Verification items for the finished model (mm, model axes). A direction names the side the tool comes from. Give positions to 0.01 mm unless a question says otherwise; leave off trailing zeros. Write each loop counter-clockwise with the first axis right and the second up, starting at its lowest first coordinate (ties: lowest second). Pieces come first, ordered by that corner, then holes. Notation, with made-up numbers: (24, -14) -> (29, -14) arc R26 ccw to (29, 18) -> close; hole circle Ø9 at (84, -29). An arc over 180 degrees is marked (long way). Answer as CSV lines item,"result". Start each with the question number.
1) Material ranges on L1, parallel to Y at x = 0, z = 0.75; L2, parallel to Y at x = -1, z = 1; L3, parallel to Z at x = 8.5, y = 3.5, recorded low to high.
2) Mould release check, pull along Y, two halves, no side actions. Record for faces 4 (the flat face through (3.647, 1.634, 6.234)), 5 (the flat face through (-1.836, -3.251, 3.847)), 6 (the flat face through (4.3, 2.4, 1.5)), 7 (the flat face through (1.836, 3.251, 3.885)): released by +Y, released by -Y, zero draft, split by the parting line, or undercut.
3) Tool access check on faces 1 (the cylindrical face through (-1.177, -3.875, 6.935)), 2 (the cylindrical face through (-3.35, -1.89, 5.49)), 3 (the flat face through (3.251, 1.836, 3.847)). Record the directions out of +Z, -Z, +X, -X, +Y, -Y that give a thin tool (end or side, any length) a straight path to the whole face; none if there is none.
4) Gauge pin test, flat ends, axial feed: pin 1 Ø3.5 at (x, y) = (0, -7) entering from +Z; pin 2 Ø3 at (y, z) = (-4, 1) entering from +X; pin 3 Ø4 at (x, z) = (4.5, 4) entering from +Y. Record the tip position at first contact, or that the pin passes through.
5) Sectioned sample at D-D on y = 7. Record the cut outline in (x, z).
6) Sectioned sample at C-C on z = 2.75. Record the cut outline in (x, y), and give its area (3 significant figures).
7) Sectioned sample at B-B on x = 0. Record the cut outline in (y, z).
8) Sectioned sample at A-A on z = 1. Record the cut outline in (x, y), and give its area (3 significant figures).
```python
from build123d import *

# Parameters (mm, degrees)
ESQUISSE1_R                  = 3
BOSS_EXTRU_1_DEPTH           = 1.5
ENL_V_MAT_EXTRU_1_DEPTH      = 16.779733838
ENL_V_MAT_EXTRU_1_DEPTH_BACK = 16.779733838
ESQUISSE4_R                  = 1.5
ENL_V_MAT_EXTRU_2_DEPTH      = 14.2
CONG_2_R                     = 0.5


with BuildPart() as part:
    # Esquisse1 → Boss.-Extru.1 (new body)
    with BuildSketch(Plane.XY):
        with BuildLine():
            Line((-4.5, 8.93028555), (-4.5, -8.93028555))
            ThreePointArc((-4.5, -8.93028555), (5.029430583, -8.643195475), (9.987487585, -0.500091723))
            ThreePointArc((9.987487585, -0.500091723), (5.455376603, 8.380863089), (-4.5, 8.93028555))
        make_face()
        with Locations(Location((0, 0, 0), (0, 0, 180))):
            Circle(ESQUISSE1_R, mode=Mode.SUBTRACT)
    extrude(amount=BOSS_EXTRU_1_DEPTH)

    # Esquisse2 → R_volution1 (revolve)
    with BuildSketch(Plane(origin=(0, 0, 0), x_dir=(0, 0, -1), z_dir=(1, 0, 0)), mode=Mode.PRIVATE) as r_volution1_sk:
        Polygon((-1.5, 4.5), (-7, 4.5), (-7, 3.669872981), (-4.5, 3), (-1.5, 3), align=None)
    revolve(r_volution1_sk.sketch.rotate(Axis((0, 0, 0), (0, 0, 1)), 90), axis=Axis((0, 0, 0), (0, 0, 1)))

    # Esquisse3 → Enl_v. mat.-Extru.1 (cut, two sides)
    with BuildSketch(Plane(origin=(0, 0, 0), x_dir=(0, 0, 1), z_dir=(0.7071067811865464, 0.7071067811865488, 0))) as enl_v_mat_extru_1_sk:
        with BuildLine():
            Line((2.5, 1), (5.232050808, 1))
            ThreePointArc((5.232050808, 1), (5.490869853, 1.034074174), (5.732050808, 1.133974596))
            Line((5.732050808, 1.133974596), (7, 1.866025404))
            Line((7, 1.866025404), (7, -1.866025404))
            Line((7, -1.866025404), (5.732050808, -1.133974596))
            ThreePointArc((5.732050808, -1.133974596), (5.490869853, -1.034074174), (5.232050808, -1))
            Line((5.232050808, -1), (2.5, -1))
            ThreePointArc((2.5, -1), (1.5, 0), (2.5, 1))
        make_face()
    extrude(amount=ENL_V_MAT_EXTRU_1_DEPTH, mode=Mode.SUBTRACT)
    extrude(enl_v_mat_extru_1_sk.sketch, amount=-ENL_V_MAT_EXTRU_1_DEPTH_BACK, mode=Mode.SUBTRACT)

    # Esquisse4 → Enl_v. mat.-Extru.2 (cut)
    with BuildSketch(Plane.XY.offset(1.5)):
        with Locations((0, -7)):
            Circle(ESQUISSE4_R)
        with Locations((0, 7)):
            Circle(ESQUISSE4_R)
        with Locations((7, 0)):
            Circle(ESQUISSE4_R)
    extrude(amount=-ENL_V_MAT_EXTRU_2_DEPTH, mode=Mode.SUBTRACT)

    # Cong_2
    cong_2_edges = [part.edges().sort_by_distance(p)[0] for p in [
        (-3.884480351, -1.245521917, 7),
        (1.245521917, 3.884480351, 7),
        (3.884480351, 1.245521917, 7),
        (-1.245521917, -3.884480351, 7),
    ]]
    fillet(cong_2_edges, radius=CONG_2_R)


solid = part.part
```
Ans:
1,L1,"y = -10 to -8.5, -5.5 to -3, 3 to 5.5, 8.5 to 10"
1,L2,"y = -9.95 to -8.12, -5.88 to -2.83, 2.83 to 5.88, 8.12 to 9.95"
1,L3,"z = 0 to 1.5"
2,face 4,"released by +Y"
2,face 5,"undercut"
2,face 6,"zero draft"
2,face 7,"undercut"
3,face 1,"+Z, -X"
3,face 2,"+Z, -Y"
3,face 3,"+Z, +Y"
4,pin 1,"stops at z = 1.5"
4,pin 2,"stops at x = 9.68"
4,pin 3,"stops at y = 2.45"
5,outline,"(-4.5, 0) -> (-1.5, 0) -> (-1.5, 1.5) -> (-4.5, 1.5) -> close; (1.5, 0) -> (7.14, 0) -> (7.14, 1.5) -> (1.5, 1.5) -> close"
6,outline,"(-3.81, -2.4) -> (-2.71, -1.29) arc R3 cw to (1.29, 2.71) -> (2.4, 3.81) arc R4.5 ccw to start; (-2.4, -3.81) arc R4.5 ccw to (3.81, 2.4) -> (2.71, 1.29) arc R3 cw to (-1.29, -2.71) -> close"
6,area,"29.3 mm²"
7,outline,"(-10, 0) -> (-8.5, 0) -> (-8.5, 1.5) -> (-10, 1.5) -> close; (-5.5, 0) -> (-3, 0) -> (-3, 4.5) -> (-3.67, 7) -> (-4.5, 7) -> (-4.5, 1.5) -> (-5.5, 1.5) -> close; (3, 0) -> (5.5, 0) -> (5.5, 1.5) -> (4.5, 1.5) -> (4.5, 7) -> (3.67, 7) -> (3, 4.5) -> close; (8.5, 0) -> (10, 0) -> (10, 1.5) -> (8.5, 1.5) -> close"
8,outline,"(-4.5, -8.93) arc R10 ccw (long way) to (-4.5, 8.93) -> close; hole circle Ø6 at (0, 0); hole circle Ø3 at (0, -7); hole circle Ø3 at (0, 7); hole circle Ø3 at (7, 0)"
8,area,"194 mm²"
